Part print with two shaded views. Sizes in mm from the minimum x, y, z corner. Round coordinates to 2 decimals unless told otherwise and drop trailing zeros. Write each loop counter-clockwise with the first axis right and the second up, starting at its lowest first coordinate (ties: lowest second). Pieces come first, ordered by that corner, then holes. Notation, with made-up numbers: (6, -15) -> (25, -15) arc R17 cw to (25, 13) -> close; hole circle Ø1 at (79.5, 17). An arc over 180 degrees is marked (long way). Return JSON: item names as keys, results as strings. Group by question number.
(1) Drill centre lines: L1, parallel to Y at x = 20, z = 11.5; L2, parallel to X at y = 64.05, z = 14.25; L3, parallel to Y at x = 29, z = 12.75. Where is each one in solid material? Low to high. Write a range as from..to.
(2) Saw through at A-A (x = 29). List the corners of the cut face in (y, z), plus the area to 3 significant figures.
(3) Saw through at B-B (y = 51.05). List the corners of the cut face in (x, z), plus the area to 3 significant figures.
(4) Saw through at D-D (y = 64.05). List the corners of the cut face in (x, z).
(5) Saw through at C-C (z = 17.75). List the corners of the cut face in (x, y).
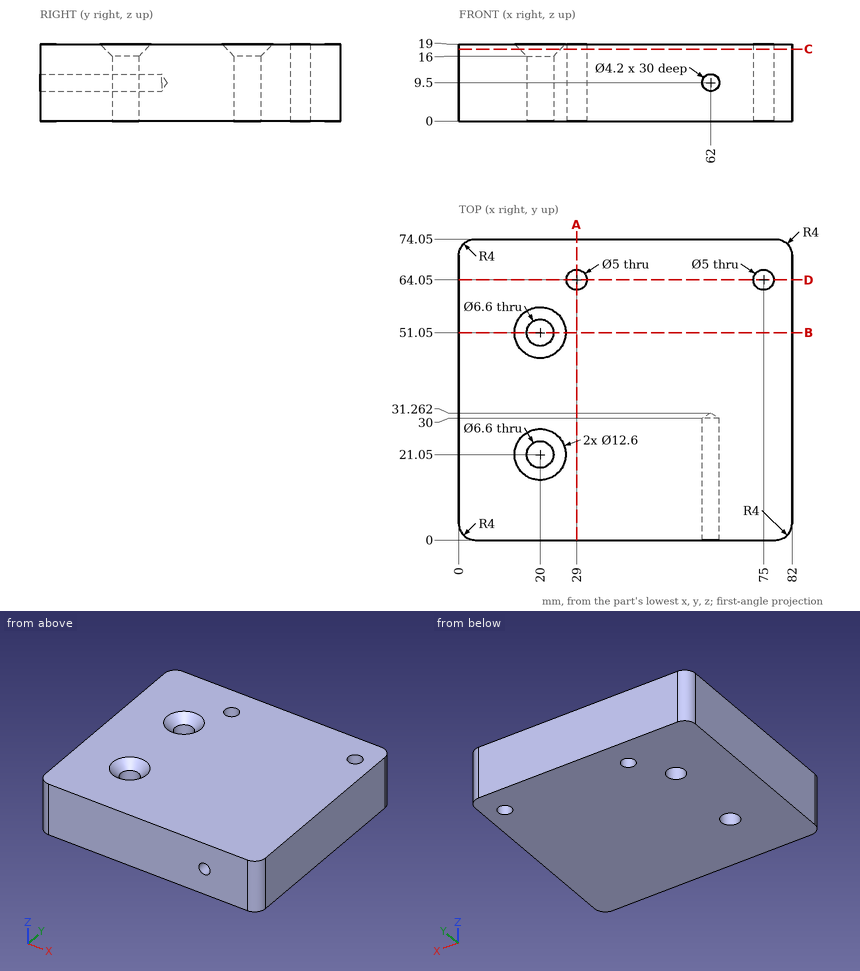
Computed values:
{
 "1": {"L1": "0..17.75, 24.35..47.75, 54.35..74.05", "L2": "0..26.5, 31.5..72.5, 77.5..82", "L3": "0..61.55, 66.55..74.05"},
 "2": {"outline": "(0, 0) -> (61.55, 0) -> (61.55, 19) -> (0, 19) -> close; (66.55, 0) -> (74.05, 0) -> (74.05, 19) -> (66.55, 19) -> close", "area": "1,310 mm2"},
 "3": {"outline": "(0, 0) -> (16.7, 0) -> (16.7, 16) -> (13.7, 19) -> (0, 19) -> close; (23.3, 0) -> (82, 0) -> (82, 19) -> (26.3, 19) -> (23.3, 16) -> close", "area": "1,420 mm2"},
 "4": {"outline": "(0, 0) -> (26.5, 0) -> (26.5, 19) -> (0, 19) -> close; (31.5, 0) -> (72.5, 0) -> (72.5, 19) -> (31.5, 19) -> close; (77.5, 0) -> (82, 0) -> (82, 19) -> (77.5, 19) -> close"},
 "5": {"outline": "(0, 4) arc R4 ccw to (4, 0) -> (78, 0) arc R4 ccw to (82, 4) -> (82, 70.05) arc R4 ccw to (78, 74.05) -> (4, 74.05) arc R4 ccw to (0, 70.05) -> close; hole circle Ø10.1 at (20, 21.05); hole circle Ø10.1 at (20, 51.05); hole circle Ø5 at (29, 64.05); hole circle Ø5 at (75, 64.05)"}
}
